Answer from the drawing. Dimensions are ordinates in mm from the lowest x, y and z of the part. A direction names the side the tool comes from. Coordinates: 2 decimals unless noted, no trailing zeros. Loops run counter-clockwise (first coordinate to the right, second up) from the corner with the lowest first, then second, coordinate; pieces in that order, holes last. Notation, with made-up numbers: (49, 32) -> (107, 32) arc R26 cw to (107, 46) -> close; hole circle Ø7 at (-19.75, 37.25). An arc over 180 degrees is marked (long way). Answer as CSV lines item,"result".
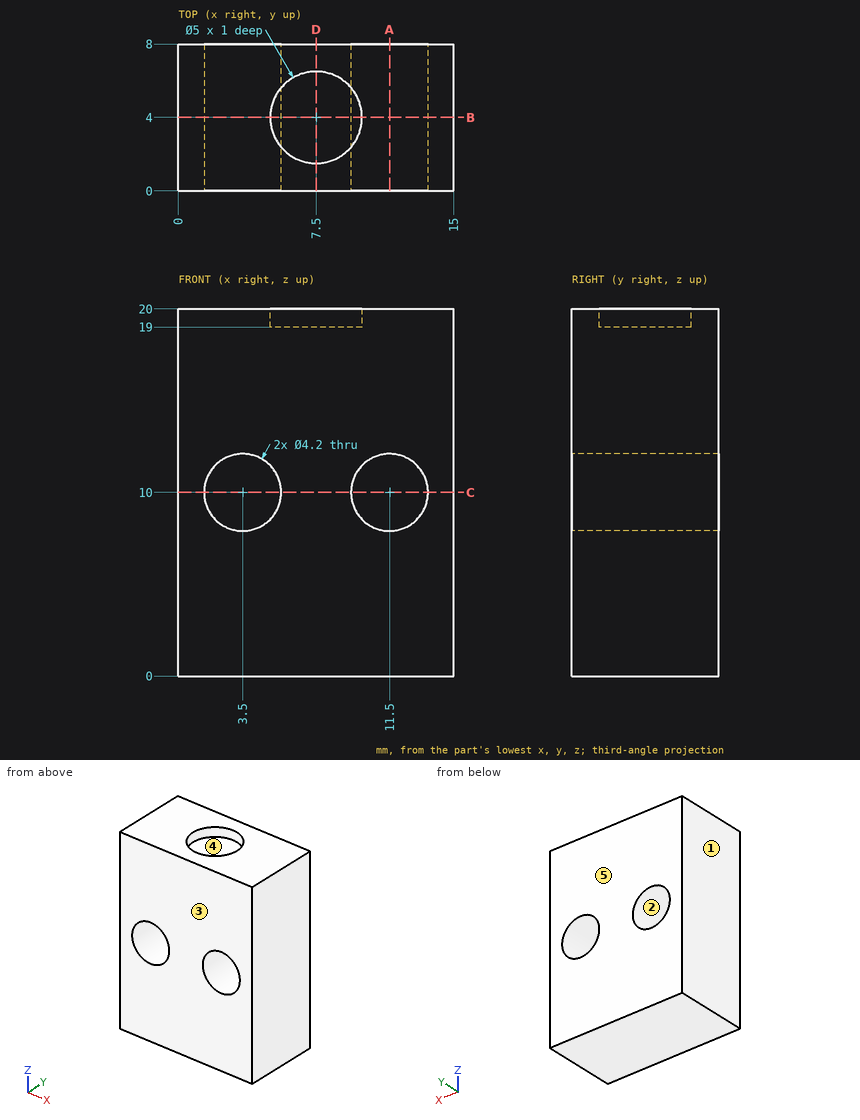
(1) A cutting plane is placed at C-C, the plane z = 10. Write down the section's boundary in (x, y), and give its area (3 significant figures).
Computed values:
outline,"(0, 0) -> (1.4, 0) -> (1.4, 8) -> (0, 8) -> close; (5.6, 0) -> (9.4, 0) -> (9.4, 8) -> (5.6, 8) -> close; (13.6, 0) -> (15, 0) -> (15, 8) -> (13.6, 8) -> close"
area,"52.8 mm2"
(2) A cutting plane is placed at A-A, the plane x = 11.5. Write down the section's boundary in (y, z).
Computed values:
outline,"(0, 0) -> (8, 0) -> (8, 7.9) -> (0, 7.9) -> close; (0, 12.1) -> (8, 12.1) -> (8, 20) -> (0, 20) -> close"
(3) A cutting plane is placed at B-B, the plane y = 4. Write down the section's boundary in (x, z), and give its area (3 significant figures).
Computed values:
outline,"(0, 0) -> (15, 0) -> (15, 20) -> (10, 20) -> (10, 19) -> (5, 19) -> (5, 20) -> (0, 20) -> close; hole circle Ø4.2 at (3.5, 10); hole circle Ø4.2 at (11.5, 10)"
area,"267 mm2"
(4) A flat-ended cylindrical pin translates along its axis: pin 1 Ø4 at (x, y) = (7.5, 4) entering from +Z. Find the tip coordinate at first contact, or state that the pin passes through.
Computed values:
pin 1,"z = 19"
(5) Which of the six approach directions +Z, -Z, +X, -X, +Y, -Y give full straight-line access (tool end or side, diameter ignored) to the marked faces 4 and 5?
Computed values:
face 4,"+Z"
face 5,"+Z, -Z, +X, -X, +Y"
(6) A cutting plane is placed at D-D, the plane x = 7.5. Write down the section's boundary in (y, z), and give its area (3 significant figures).
Computed values:
outline,"(0, 0) -> (8, 0) -> (8, 20) -> (6.5, 20) -> (6.5, 19) -> (1.5, 19) -> (1.5, 20) -> (0, 20) -> close"
area,"155 mm2"
(7) For a pull along X with two mould halves and no side action, classify the marked faces 1, 2 and 3 as pulls with the +X half, pulls with the -X half, needs draft (parallel to the pull), parting line crosses it, or undercut.
Computed values:
face 1,"pulls with the -X half"
face 2,"undercut"
face 3,"needs draft"
(8) Consider line 1 along Y through (x, z) = (7.5, 19.55); line 2 along X through (y, z) = (1.5, 11.5); line 3 along Z through (x, y) = (11.5, 2.75). Determine where each line is inside the solid, lowest interval first.
Computed values:
line 1,"0 to 1.5, 6.5 to 8"
line 2,"0 to 2.03, 4.97 to 10.03, 12.97 to 15"
line 3,"0 to 7.9, 12.1 to 20"
